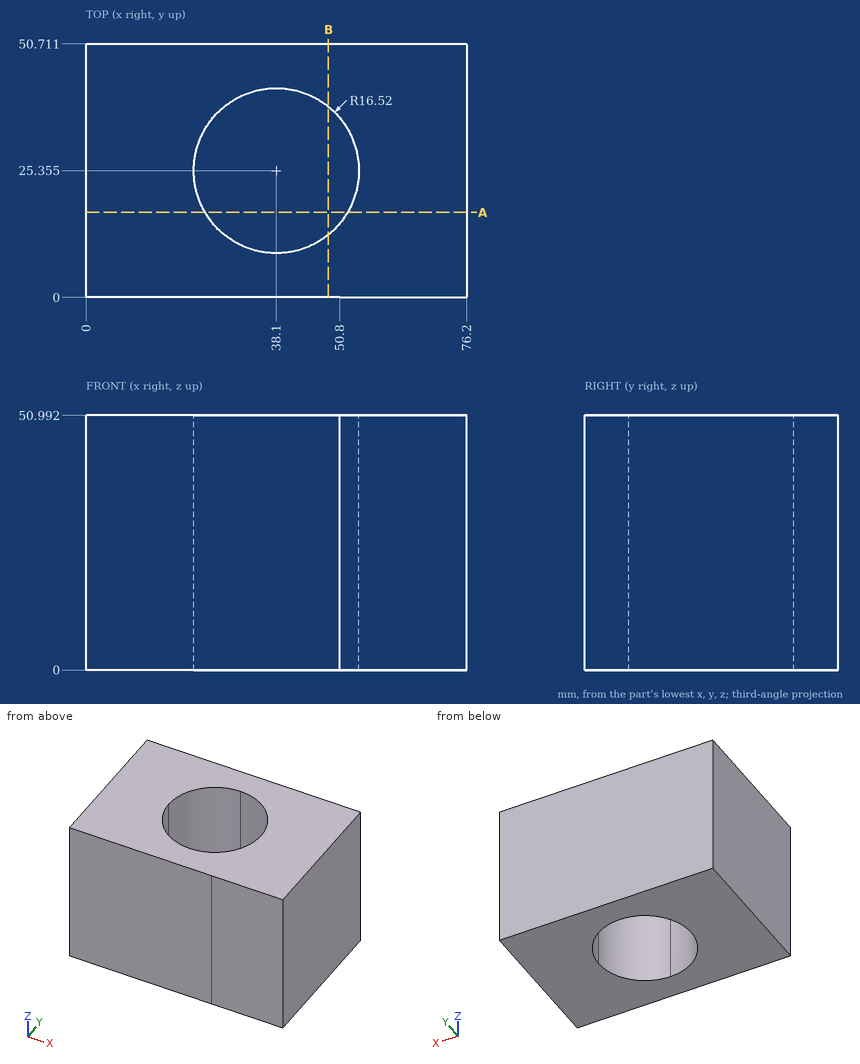
Study the drawing (mm; zero at the part's minimum x, y, z) and answer. Coordinates: 2 decimals unless noted, no trailing zeros. Loops run counter-clockwise (first coordinate to the right, second up) from the corner with the lowest first, then second, coordinate; pieces in that order, holes last. Notation, with made-up numbers: M -38,67 L 6,67 A28 cw 6,96 Z; hole C 37,50.5 d1. An arc over 180 degrees is marked long. Answer in a Markdown table with one row per item.
1) Find section B-B (x = 48.5). Determine the outline of the cut face in (y, z), then the cut area to 3 significant figures.
Answers below:
| item | result |
|---|---|
| outline | M 0,0 L 12.52,0 L 12.52,50.99 L 0,50.99 Z; M 38.19,0 L 50.71,0 L 50.71,50.99 L 38.19,50.99 Z |
| area | 1,280 mm^2 |
2) Find the intervals of material crossed by probe 1 along X at (y, z) = (25, 45); probe 2 along X at (y, z) = (31.5, 32) (1 decimal); probe 3 along Y at (x, z) = (33, 31), in increasing order.
Answers below:
| item | result |
|---|---|
| probe 1 | 0 to 21.58, 54.62 to 76.2 |
| probe 2 | 0 to 22.8, 53.4 to 76.2 |
| probe 3 | 0 to 9.64, 41.07 to 50.71 |
3) Find section A-A (y = 17). Determine the outline of the cut face in (x, z).
Answers below:
| item | result |
|---|---|
| outline | M 0,0 L 23.85,0 L 23.85,50.99 L 0,50.99 Z; M 52.35,0 L 76.2,0 L 76.2,50.99 L 52.35,50.99 Z |
